For this review, take the finished solid that the model builds, in its own axes (mm). Face numbers are marked on the shaded views. A direction names the side the tool comes from. Coordinates: 2 decimals unless noted, no trailing zeros. Order: outer loops, then holes, each group sorted by start corner. A loop starts at its lowest first (then second) coordinate and runs counter-clockwise, first axis right, second up. Notation, with made-up numbers: (-9.5, 61) -> (17.5, 61) arc R35 ccw to (17.5, 93) -> close; hole circle Ø3 at (-23, 72). An arc over 180 degrees is marked (long way). Return JSON: item names as keys, results as strings. Group by question number.
Item 1: Take a section at D-D (y = 23). Write out the cut boundary in (x, z).
Item 2: Take a section at C-C (x = 0). Write out the cut boundary in (y, z), then the cut area to 3 significant figures.
Item 3: Take a section at A-A (z = -10). Write out the cut boundary in (x, y).
Item 4: Insertion check: pin 1 (4 mm diameter, centred on x = 19.5, z = -7.5, fed in from -Y); pin 2 (7 mm diameter, centred on x = 24.62, z = 9, fed in from -Y); pin 3 (6 mm diameter, centred on x = 10.5, z = 2, fed in from +Y). Each pin has a flat end and moves straight along its axis. Give the tip position at first contact, or say it passes through.
Item 5: For line 1 along X through (y, z) = (2.5, -10); line 2 along X through (y, z) = (9.5, -10); line 3 along Y through (x, z) = (27, 2), list the stretches that pass through material, from the lowest coordinate up.
Item 6: Machinability: for the marked faces 1, 2 and 3, which of the approach directions +Z, -Z, +X, -X, +Y, -Y give a long, thin tool a straight path to every point of the face, cutting with its end or side? Answer none if there is none.
Item 7: Take a section at B-B (y = 9). Write out the cut boundary in (x, z).
```python
from build123d import *

# Parameters (mm, degrees)
SKETCH1_W                     = 34
SKETCH1_H                     = 27
BOSS_EXTRUDE1_DEPTH           = 11
SKETCH2_R                     = 20.25
SKETCH2_R_2                   = 16.25
MOTOR_CLAMP_BAND_DEPTH        = 20
FILLET4_R                     = 5
SKETCH7_W                     = 15
SKETCH7_H                     = 15
BOSS_EXTRUDE3_DEPTH           = 20
FILLET5_R                     = 5
CBORE_FOR_M3_SHCS1_AT_2_COUNT = 2
CBORE_FOR_M3_SHCS1_AT_2_PITCH = 15
CBORE_FOR_M3_SHCS1_AT_3_COUNT = 2
CBORE_FOR_M3_SHCS1_AT_3_PITCH = 25
CBORE_FOR_M3_SHCS1_AT_4_COUNT = 2
CBORE_FOR_M3_SHCS1_AT_4_PITCH = 20
EXTENDED_START                = 15
SKETCH6_R                     = 3.25
EXTENDED_COUNTERBORE_1_DEPTH  = 15
M4_CLEARANCE_HOLE1_D          = 4.5
CUT_EXTRUDE2_DEPTH            = 3
SKETCH14_W                    = 15.007694129
SKETCH14_H                    = 1
CUT_EXTRUDE3_DEPTH            = 65.465591597
FILLET3_R                     = 5


with BuildPart() as part:
    # Sketch1 → Boss-Extrude1 (new body)
    with BuildSketch(Plane(origin=(0, 0, 0), x_dir=(1, 0, 0), z_dir=(0, 1, 0))):
        Rectangle(SKETCH1_W, SKETCH1_H)
    extrude(amount=BOSS_EXTRUDE1_DEPTH)

    # Sketch2 → Motor Clamp Band (add)
    with BuildSketch(Plane.XY.offset(13.5)):
        with Locations((0, 29.25)):
            Circle(SKETCH2_R)
        with Locations((0, 29.25)):
            Circle(SKETCH2_R_2, mode=Mode.SUBTRACT)
    extrude(amount=-MOTOR_CLAMP_BAND_DEPTH)

    # Fillet4
    # the kernel refuses this fillet: 5 mm, written as the material it adds along each edge
    with BuildSketch(Plane(origin=(8.774964387, 11, -6.5), x_dir=(0.7657018852259857, 0.6431956335061453, 0), z_dir=(0, 0, 1))) as fillet4_piece_1:
        with BuildLine():
            CenterArc((11.27796375, -4.843969922), FILLET4_R, 104.351347878, 80.770115484)
            Line((6.297925275, -5.290306991), (6.198324505, -5.299233733))
            ThreePointArc((6.198324505, -5.299233733), (3.084643074, -2.721723684), (-0.064319563, -0.076570189))
            Line((-0.064319563, -0.076570189), (0.024786734, 0.096879398))
            ThreePointArc((0.024786734, 0.096879398), (5.019313537, -0.531921816), (10.013840341, 0.096879398))
            Line((10.013840341, 0.096879398), (10.038627075, 0))
        make_face()
    extrude(amount=20)

    # Sketch7 → Boss-Extrude3 (add)
    with BuildSketch(Plane.XY.offset(13.5)):
        with Locations((23.75, 26.75)):
            Rectangle(SKETCH7_W, SKETCH7_H)
    extrude(amount=-BOSS_EXTRUDE3_DEPTH)

    # Fillet5
    # the kernel refuses this fillet: 5 mm, written as the material it adds along each edge
    with BuildSketch(Plane(origin=(-8.774964387, 11, -6.5), x_dir=(-1, 0, 0), z_dir=(0, 0, 1))) as fillet5_piece_1:
        with BuildLine():
            CenterArc((11.751178408, -3.544900138), FILLET5_R, 134.848011946, 80.770115484)
            Line((7.686595676, -6.456801101), (7.605304021, -6.51503912))
            ThreePointArc((7.605304021, -6.51503912), (4.185427628, -2.821107013), (-0.043333157, -0.090123457))
            Line((-0.043333157, -0.090123457), (0, 0.1))
            ThreePointArc((0, 0.1), (4.112517806, 0.1), (8.154512757, 0.070898003))
            Line((8.154512757, 0.070898003), (8.225035613, 0))
        make_face()
    extrude(amount=20)

    # Sketch4 → CBORE for M3 SHCS1 (revolve, cut)
    with BuildSketch(Plane(origin=(7.5, 11, -10), x_dir=(0, 0, 1), z_dir=(1, 0, 0))):
        Polygon((0, 0), (0, 11), (1.7, 11), (1.7, 3), (3.25, 3), (3.25, 0), align=None)
    cbore_for_m3_shcs1 = revolve(axis=Axis((7.5, 17.35, -10), (0, -1, 0)), mode=Mode.SUBTRACT)

    # CBORE for M3 SHCS1 at 2: CBORE for M3 SHCS1 ×2
    with Locations(*[(-i * CBORE_FOR_M3_SHCS1_AT_2_PITCH, 0, 0) for i in range(1, CBORE_FOR_M3_SHCS1_AT_2_COUNT)]):
        add(cbore_for_m3_shcs1, mode=Mode.SUBTRACT)

    # CBORE for M3 SHCS1 at 3: CBORE for M3 SHCS1 ×2
    with Locations(*[Vector(-0.5999999999999989, 0, 0.8000000000000009) * (i * CBORE_FOR_M3_SHCS1_AT_3_PITCH) for i in range(1, CBORE_FOR_M3_SHCS1_AT_3_COUNT)]):
        add(cbore_for_m3_shcs1, mode=Mode.SUBTRACT)

    # CBORE for M3 SHCS1 at 4: CBORE for M3 SHCS1 ×2
    with Locations(*[(0, 0, i * CBORE_FOR_M3_SHCS1_AT_4_PITCH) for i in range(1, CBORE_FOR_M3_SHCS1_AT_4_COUNT)]):
        add(cbore_for_m3_shcs1, mode=Mode.SUBTRACT)

    # Sketch6 → Extended CounterBore 1 (cut)
    with BuildSketch(Plane(origin=(0, 11, 0), x_dir=(1, 0, 0), z_dir=(0, 1, 0)).offset(EXTENDED_START)):
        with Locations(Location((7.5, -10, 0), (0, 0, 270))):
            Circle(SKETCH6_R)
        with Locations(Location((-7.5, -10, 0), (0, 0, 270))):
            Circle(SKETCH6_R)
    extrude(amount=-EXTENDED_COUNTERBORE_1_DEPTH, mode=Mode.SUBTRACT)

    # M4 Clearance Hole1 (through all)
    with Locations(Plane(origin=(0, 34.25, 0), x_dir=(-1, 0, 0), z_dir=(0, 1, 0))):
        with Locations((-24.623009453, -2), (-24.623009453, 9)):
            Hole(M4_CLEARANCE_HOLE1_D / 2)

    # Sketch13 → Cut-Extrude2 (cut)
    with BuildSketch(Plane.XZ.offset(-19.25)):
        Polygon((24.623009453, 12.954849344), (21.198009453, 10.977424672), (21.198009453, 7.022575328), (24.623009453, 5.045150656), (28.048009453, 7.022575328), (28.048009453, 10.977424672), align=None)
        Polygon((28.048009453, -0.022575328), (24.623009453, 1.954849344), (21.198009453, -0.022575328), (21.198009453, -3.977424672), (24.623009453, -5.954849344), (28.048009453, -3.977424672), align=None)
    extrude(amount=-CUT_EXTRUDE2_DEPTH, mode=Mode.SUBTRACT)

    # Sketch14 → Cut-Extrude3 (cut, through all)
    with BuildSketch(Plane.XY.offset(13.5)):
        with Locations((23.746152936, 29.25)):
            Rectangle(SKETCH14_W, SKETCH14_H)
    extrude(amount=-CUT_EXTRUDE3_DEPTH, mode=Mode.SUBTRACT)

    # Fillet3
    # the kernel refuses this fillet: 5 mm, written as the material it adds along each edge
    with BuildSketch(Plane(origin=(17.608591653, 19.25, -6.5), x_dir=(-0.5388484844645524, -0.8424027010820033, 0), z_dir=(0, 0, 1))) as fillet3_piece_1:
        with BuildLine():
            CenterArc((2.762959446, 4.959604744), FILLET3_R, 212.605284551, 50.106677373)
            Line((-1.44905406, 2.265362322), (-1.53329433, 2.211477474))
            Line((-1.53329433, 2.211477474), (-0.08424027, -0.053884848))
            Line((-0.08424027, -0.053884848), (0.00525598, -0.099861778))
            ThreePointArc((0.00525598, -0.099861778), (1.064335915, -0.072010015), (2.115986078, -0.099192095))
            Line((2.115986078, -0.099192095), (2.12867183, 0))
        make_face()
    extrude(amount=20)


solid = part.part
```
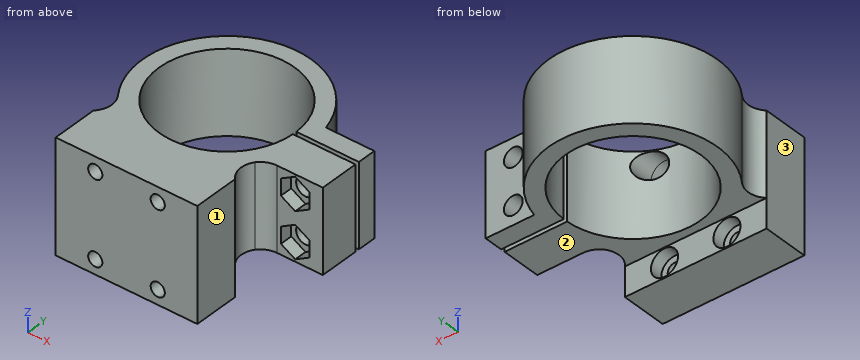
Findings below:
{
 "1": {"outline": "(-19.26, -6.5) -> (-15, -6.5) -> (-15, 13.5) -> (-19.26, 13.5) -> close; (15, -6.5) -> (31.25, -6.5) -> (31.25, 13.5) -> (15, 13.5) -> close; hole circle Ø4.5 at (24.62, -2); hole circle Ø4.5 at (24.62, 9)"},
 "2": {"outline": "(0, -13.5) -> (11, -13.5) -> (11, -6.5) -> (13, -6.5) -> (13, 13.5) -> (0, 13.5) -> close; (45.5, -6.5) -> (49.5, -6.5) -> (49.5, 13.5) -> (45.5, 13.5) -> close", "area": "417 mm2"},
 "3": {"outline": "(-17, 0) -> (-9.2, 0) -> (-9.2, 8) -> (-10.75, 8) -> (-10.75, 11) -> (-17, 11) -> close; (-5.8, 0) -> (5.8, 0) -> (5.8, 8) -> (4.25, 8) -> (4.25, 11) -> (-4.25, 11) -> (-4.25, 8) -> (-5.8, 8) -> close; (9.2, 0) -> (17, 0) -> (17, 11) -> (10.75, 11) -> (10.75, 8) -> (9.2, 8) -> close"},
 "4": {"pin 1": "stops at y = 18.56", "pin 2": "stops at y = 19.25", "pin 3": "stops at y = 48.06"},
 "5": {"line 1": "x = -17 to -9.2, -5.8 to 5.8, 9.2 to 17", "line 2": "x = -17 to -10.75, -4.25 to 4.25, 10.75 to 17", "line 3": "y = 19.25 to 28.75, 29.75 to 34.25"},
 "6": {"face 1": "+Z, -Z, +X, -Y", "face 2": "-Z, +X, -X, +Y", "face 3": "+Z, -Z, -X, -Y"},
 "7": {"outline": "(-17, -13.5) -> (17, -13.5) -> (17, 13.5) -> (-17, 13.5) -> close; hole circle Ø6.5 at (-7.5, -10); hole circle Ø6.5 at (-7.5, 10); hole circle Ø6.5 at (7.5, -10); hole circle Ø6.5 at (7.5, 10)"}
}
